Input: part model. Units: mm. Frame: model coordinates. Face numbers are marked on the shaded views. A direction names the side the tool comes from. Coordinates: 2 decimals unless noted, no trailing zeros. Loops run counter-clockwise (first coordinate to the right, second up) from the corner with the lowest first, then second, coordinate; pieces in that order, holes last.
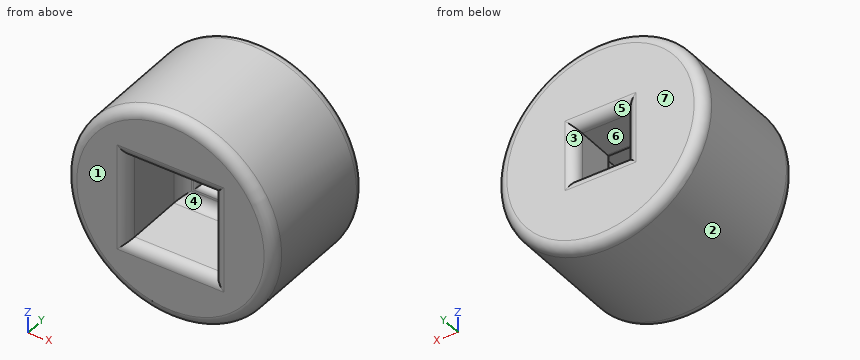
```python
from build123d import *

# Parameters (mm, degrees)
F0_R     = 20
F1_DEPTH = 25
F2_W     = 16.5
F2_H     = 16.5
F3_DEPTH = 15
F4_W     = 9.7
F4_H     = 9.7
F5_DEPTH = 25
F6_R     = 2
F7_R     = 1


with BuildPart() as f1:
    # F0 (on Front) → F1 (new body)
    with BuildSketch(Plane.XZ):
        Circle(F0_R)
    extrude(amount=F1_DEPTH)

    # F2 (on face) → F3 (cut)
    with BuildSketch(Plane.XZ.offset(25)):
        Rectangle(F2_W, F2_H)
    extrude(amount=-F3_DEPTH, mode=Mode.SUBTRACT)

    # F4 (on face) → F5 (cut)
    with BuildSketch(Plane(origin=(0, 0, 0), x_dir=(-1, 0, 0), z_dir=(0, 1, 0))):
        Rectangle(F4_W, F4_H)
    extrude(amount=-F5_DEPTH, mode=Mode.SUBTRACT)

    # F6
    f6_edges = [f1.edges().sort_by_distance(p)[0] for p in [
        (0, -10, -8.25),
        (-8.25, -10, 0),
        (8.25, -10, 0),
        (0, -10, 8.25),
        (-20, -25, 0),
        (0, -25, 8.25),
        (-8.25, -25, 0),
        (0, -25, -8.25),
        (8.25, -25, 0),
        (-20, 0, 0),
        (-4.85, 0, 0),
        (0, 0, -4.85),
        (4.85, 0, 0),
        (0, 0, 4.85),
    ]]
    fillet(f6_edges, radius=F6_R)

    # F7
    f7_edges = [f1.edges().sort_by_distance(p)[0] for p in [
        (0, -10, -4.85),
        (-4.85, -10, 0),
        (0, -10, 4.85),
        (4.85, -10, 0),
    ]]
    fillet(f7_edges, radius=F7_R)


solid = f1.part
```
Item 1: Section query A-A (x = 0). Output: boundary loops of the cut face in (y, z), then the cut area to 3 significant figures.
Result:
outline: (-25, -18) arc R2 ccw to (-23, -20) - (-2, -20) arc R2 ccw to (0, -18) - (0, -6.85) arc R2 ccw to (-2, -4.85) - (-9, -4.85) arc R1 ccw to (-10, -5.85) - (-10, -6.25) arc R2 cw to (-12, -8.25) - (-23, -8.25) arc R2 ccw to (-25, -10.25) - close; (-25, 10.25) arc R2 ccw to (-23, 8.25) - (-12, 8.25) arc R2 cw to (-10, 6.25) - (-10, 5.85) arc R1 ccw to (-9, 4.85) - (-2, 4.85) arc R2 ccw to (0, 6.85) - (0, 18) arc R2 ccw to (-2, 20) - (-23, 20) arc R2 ccw to (-25, 18) - close
area: 650 mm2
Item 2: Mould query, pull axis X, two halves, no side actions, for the marked faces 1, 2 and 3. Classes: +X half, -X half, draft (parallel to the pull), parting line (faces both ways), or undercut.
Result:
face 1: draft
face 2: parting line
face 3: undercut
Item 3: Section query C-C (y = -20.75). Output: boundary loops of the cut face in (x, z).
Result:
outline: circle Ø40 at (0, 0); hole (-8.25, -8.25) - (8.25, -8.25) - (8.25, 8.25) - (-8.25, 8.25) - close
Item 4: Section query B-B (z = 0). Output: boundary loops of the cut face in (x, y), then the cut area to 3 significant figures.
Result:
outline: (-20, -23) arc R2 ccw to (-18, -25) - (-10.25, -25) arc R2 ccw to (-8.25, -23) - (-8.25, -12) arc R2 cw to (-6.25, -10) - (-5.85, -10) arc R1 ccw to (-4.85, -9) - (-4.85, -2) arc R2 ccw to (-6.85, 0) - (-18, 0) arc R2 ccw to (-20, -2) - close; (4.85, -9) arc R1 ccw to (5.85, -10) - (6.25, -10) arc R2 cw to (8.25, -12) - (8.25, -23) arc R2 ccw to (10.25, -25) - (18, -25) arc R2 ccw to (20, -23) - (20, -2) arc R2 ccw to (18, 0) - (6.85, 0) arc R2 ccw to (4.85, -2) - close
area: 650 mm2
Item 5: Reachability of the marked faces 4, 5, 6 and 7 from +Z, -Z, +X, -X, +Y, -Y: full face, straight path, thin tool, end or side. Return the list, or none.
Result:
face 4: -Y
face 5: +Y
face 6: +Y, -Y
face 7: +Z, -Z, +X, -X, +Y
Item 6: Contact query for flat-ended pins moving along their axis: P1, Ø3.5, axis at x = 1.5, y = -19, coming from the +Z side; P2, Ø12, axis at x = -2.5, y = -19.5, coming from the -Z side; P3, Ø1.5, axis at x = -9, y = -20, coming from the +Z side. Output: stop coordinate, or through.
Result:
P1: stops at z = 20
P2: stops at z = -20
P3: stops at z = 18.22
Item 7: Line query: L1, parallel to X at y = -12.75, z = -4; L2, parallel to Y at x = 1.5, z = -5.5; L3, parallel to X at y = -7, z = 14. Output: solid intervals per line, ascending.
Result:
L1: x = -19.6 to -8.25, 8.25 to 19.6
L2: y = -9.94 to -0.52
L3: x = -14.28 to 14.28
